Model file for the job. Use its own axes, mm. Face numbers are marked on the shaded views. A direction names the side the tool comes from. Coordinates: 2 decimals unless noted, no trailing zeros. Order: outer loops, then holes, each group sorted by start corner. A loop starts at its lowest first (then second) coordinate and runs counter-clockwise, first axis right, second up. Notation, with made-up numbers: (-8, 42.25) -> (33, 42.25) arc R25 cw to (33, 68.25) -> close; hole circle Ø9 at (20, -39). An arc over 180 degrees is marked (long way). Return JSON: item names as keys, results as strings. Group by question number.
1) Probe line 1 (Y direction, x = -8.1, z = 0); line 2 (Z direction, x = 7.2, y = 21); line 3 (Y direction, x = -1, z = -5). List the from-to ranges inside material, lowest first.
2) Cut at C-C (y = 21.75). Write the cut outline in (x, z), and give its area (3 significant figures).
3) Flat gauge pins, fed straight in: pin 1 (2 mm diameter, centred on y = 20, z = 1, fed in from -X); pin 2 (1.5 mm diameter, centred on x = 1, y = 10.5, fed in from +Z); pin 3 (4 mm diameter, centred on x = -6.5, y = 15, fed in from -Z). Where does each tip first touch, or does it go through?
4) Pull direction Y, two halves, no side cores. Call the marked faces 4, 5, 6 and 7: +Y half, -Y half, draft (parallel to the pull), parting line (faces both ways), or undercut.
5) Cut at D-D (z = 5). Write the cut outline in (x, y), and give its area (3 significant figures).
6) Which spindle directions (+Z, -Z, +X, -X, +Y, -Y) get a long thin tool onto all of the face, cutting with end or side? Do the marked faces 1, 2 and 3. Say none if no direction does.
7) Cut at B-B (z = 0). Write the cut outline in (x, y).
8) Cut at A-A (x = 0). Write the cut outline in (y, z).
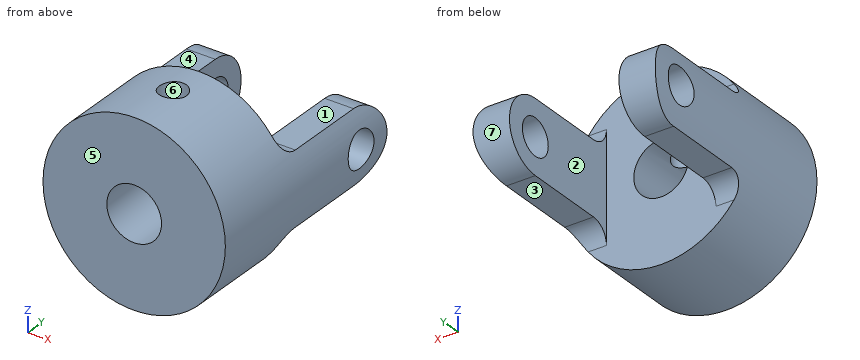
from build123d import *

# Parameters (mm, degrees)
SKETCH_1_W          = 20
SKETCH_1_H          = 20
EXTRUDE_1_DEPTH     = 10
SKETCH_2_R          = 2
EXTRUDE_2_DEPTH     = 10
SKETCH_2_2_R        = 2
CUT_EXTRUDE_1_DEPTH = 6
SKETCH_4_OUTSIDE_W  = 29.55
SKETCH_4_OUTSIDE_H  = 29.55
SKETCH_4_OUTSIDE_R  = 10
CUT_EXTRUDE_2_DEPTH = 26
SKETCH_5_R          = 3
CUT_EXTRUDE_3_DEPTH = 26.0000001
SKETCH_6_R          = 1.5
CUT_EXTRUDE_4_DEPTH = 11.0000001
FILLET_1_R          = 2


with BuildPart() as part:
    # 草圖1 → 填料-伸長1 (new body)
    with BuildSketch(Plane(origin=(0, 0, 0), x_dir=(1, 0, 0), z_dir=(0, 1, 0))):
        Rectangle(SKETCH_1_W, SKETCH_1_H)
    extrude(amount=EXTRUDE_1_DEPTH)

    # 草圖2 → 填料-伸長2 (add, symmetric)
    with BuildSketch(Plane(origin=(0, 0, 0), x_dir=(0, 0, -1), z_dir=(1, 0, 0))):
        with BuildLine():
            Line((4, 10), (4, 21))
            ThreePointArc((4, 21), (0, 25), (-4, 21))
            Line((-4, 21), (-4, 10))
            Line((-4, 10), (4, 10))
        make_face()
        with Locations((0, 21)):
            Circle(SKETCH_2_R, mode=Mode.SUBTRACT)
    extrude(amount=EXTRUDE_2_DEPTH, both=True)

    # 草圖2<2> → 除料-伸長1 (cut, symmetric)
    with BuildSketch(Plane(origin=(0, 0, 0), x_dir=(0, 0, -1), z_dir=(1, 0, 0))):
        with BuildLine():
            Line((4, 10), (4, 21))
            ThreePointArc((4, 21), (0, 25), (-4, 21))
            Line((-4, 21), (-4, 10))
            Line((-4, 10), (4, 10))
        make_face()
        with Locations((0, 21)):
            Circle(SKETCH_2_2_R, mode=Mode.SUBTRACT)
    extrude(amount=CUT_EXTRUDE_1_DEPTH, both=True, mode=Mode.SUBTRACT)

    # 草圖4 outside → 除料-伸長2 (cut, through all)
    with BuildSketch(Plane(origin=(0, 0, 0), x_dir=(1, 0, 0), z_dir=(0, 1, 0))):
        Rectangle(SKETCH_4_OUTSIDE_W, SKETCH_4_OUTSIDE_H)
        Circle(SKETCH_4_OUTSIDE_R, mode=Mode.SUBTRACT)
    extrude(amount=CUT_EXTRUDE_2_DEPTH, mode=Mode.SUBTRACT)

    # 草圖5 → 除料-伸長3 (cut, through all)
    with BuildSketch(Plane.XZ):
        Circle(SKETCH_5_R)
    extrude(amount=-CUT_EXTRUDE_3_DEPTH, mode=Mode.SUBTRACT)

    # 草圖6 → 除料-伸長4 (cut, through all)
    with BuildSketch(Plane.XY):
        with Locations((0, 6)):
            Circle(SKETCH_6_R)
    extrude(amount=CUT_EXTRUDE_4_DEPTH, mode=Mode.SUBTRACT)

    # 圓角1
    fillet_1_edges = [part.edges().sort_by_distance(p)[0] for p in [
        (-7.582575695, 10, 4),
        (-7.582575695, 10, -4),
        (7.582575695, 10, 4),
        (7.582575695, 10, -4),
    ]]
    fillet(fillet_1_edges, radius=FILLET_1_R)


solid = part.part
Answers below:
{
 "1": {"line 1": "y = 0 to 19, 23 to 25", "line 2": "z = -4 to -2, 2 to 4", "line 3": "y = 0 to 10"},
 "2": {"outline": "(-9.83, -1.85) arc R10 ccw to (-9.2, -3.93) -> (-6, -3.93) -> (-6, -1.85) -> close; (-9.83, 1.85) -> (-6, 1.85) -> (-6, 3.93) -> (-9.2, 3.93) arc R10 ccw to start; (6, -3.93) -> (9.2, -3.93) arc R10 ccw to (9.83, -1.85) -> (6, -1.85) -> close; (6, 1.85) -> (9.83, 1.85) arc R10 ccw to (9.2, 3.93) -> (6, 3.93) -> close", "area": "29.5 mm^2"},
 "3": {"pin 1": "stops at x = -9.98", "pin 2": "stops at z = 9.99", "pin 3": "stops at z = -4"},
 "4": {"face 4": "draft", "face 5": "-Y half", "face 6": "undercut", "face 7": "+Y half"},
 "5": {"outline": "(-8.66, 0) -> (8.66, 0) -> (8.66, 10.27) -> (6, 10.27) -> (6, 10) -> (-6, 10) -> (-6, 10.27) -> (-8.66, 10.27) -> close; hole circle Ø3 at (0, 6)", "area": "168 mm^2"},
 "6": {"face 1": "+Z, +X, -X, +Y", "face 2": "+Z, -Z, +Y", "face 3": "-Z, +X, -X, +Y"},
 "7": {"outline": "(-10, 0) -> (-3, 0) -> (-3, 10) -> (-6, 10) -> (-6, 19) -> (-10, 19) -> close; (-10, 23) -> (-6, 23) -> (-6, 25) -> (-10, 25) -> close; (3, 0) -> (10, 0) -> (10, 19) -> (6, 19) -> (6, 10) -> (3, 10) -> close; (6, 23) -> (10, 23) -> (10, 25) -> (6, 25) -> close"},
 "8": {"outline": "(0, -10) -> (10, -10) -> (10, -3) -> (0, -3) -> close; (0, 3) -> (4.5, 3) -> (4.5, 10) -> (0, 10) -> close; (7.5, 3) -> (10, 3) -> (10, 10) -> (7.5, 10) -> close"}
}
